Verification items for the finished model (mm, model axes). Face numbers are marked on the shaded views. A direction names the side the tool comes from. Give positions to 0.01 mm unless a question says otherwise; leave off trailing zeros. Write each loop counter-clockwise with the first axis right and the second up, starting at its lowest first coordinate (ties: lowest second). Pieces come first, ordered by that corner, then holes. Notation, with made-up numbers: (-25.75, 79.25) - (-9.75, 79.25) arc R36 ccw to (-9.75, 114.25) - close; hole circle Ø11 at (27, 70.25). An arc over 180 degrees is marked (long way). Answer as a JSON object with one key per item and string values. Group by question number.
Item 1: Scan lines: line 1 along Y through (x, z) = (1312.5, 29); line 2 along X through (y, z) = (-642, 140). Record each from-to range of solid material in increasing order. Write a range as [from, to].
Item 2: Tool access check on the marked faces 1 and 2. Record the directions out of +Z, -Z, +X, -X, +Y, -Y that give a thin tool (end or side, any length) a straight path to the whole face; none if there is none.
Item 3: Sectioned sample at C-C, the plane x = 1124.5. Record the boundary of the cut face in (y, z).
Item 4: Go/stop test with a flat-tipped pin: pin 1 (1.5 mm diameter, centred on y = -639.5, z = 38, fed in from +X). Record where the tip stops, or that it passes through.
Item 5: Sectioned sample at B-B, the plane z = 73.5. Record the boundary of the cut face in (x, y).
Item 6: Sectioned sample at A-A, the plane y = -674.5. Record the boundary of the cut face in (x, z), and give its area (3 significant figures).
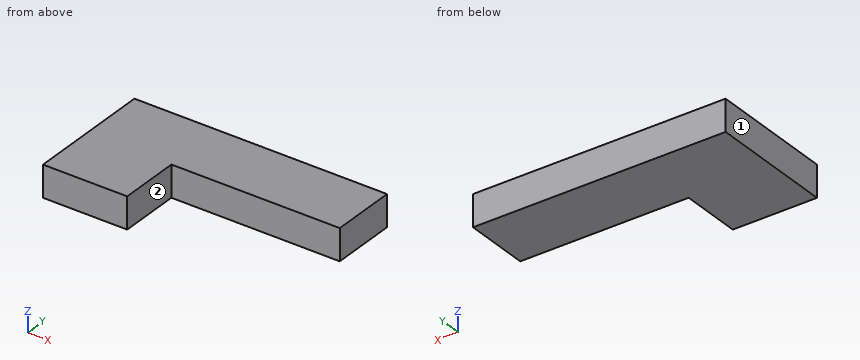
Autodesk Inventor part; units mm, degrees
ref_plane "YZ Plane" through (0, 0, 0) normal (1, 0, 0) x (0, 1, 0)
ref_plane "XZ Plane" through (0, 0, 0) normal (0, 1, 0) x (-1, 0, 0)
ref_plane "XY Plane" through (0, 0, 0) normal (0, 0, 1) x (1, 0, 0)
sketch "Sketch1" plane through (0, 0, 0) normal (0, 0, 1) x (1, 0, 0)
  line L0 (0, 0) -> (1524, 0)
  line L1 (1524, 0) -> (1524, -393.7)
  line L2 (1524, -393.7) -> (508, -393.7)
  line L3 (0, -393.7) -> (0, 0)
  line L4 (0, 0) -> (928.4892, 0)
  line L5 (420.4892, -393.7) -> (508, -393.7)
  line L6 (0, -393.7) -> (0, 0)
  line L7 (0, 0) -> (508, 0)
  line L8 (508, -393.7) -> (508, -762)
  line L9 (508, -762) -> (0, -762)
  line L10 (0, -762) -> (0, 0)
  dimension "d0" = 393.7
  dimension "d1" = 1524
  dimension "d2" = 762
  dimension "d3" = 508
extrude "Extrusion1" add sketch "Sketch1" along normal blind 190.5
properties part number "laser-enclosure"
Geometry check:
{
 "1": {"line 1": "[-393.7, 0]", "line 2": "[0, 508]"},
 "2": {"face 1": "+Z, -Z, -X, +Y, -Y", "face 2": "+Z, -Z, +X, -Y"},
 "3": {"outline": "(-393.7, 0) - (0, 0) - (0, 190.5) - (-393.7, 190.5) - close"},
 "4": {"pin 1": "x = 508"},
 "5": {"outline": "(0, -762) - (508, -762) - (508, -393.7) - (1524, -393.7) - (1524, 0) - (0, 0) - close"},
 "6": {"outline": "(0, 0) - (508, 0) - (508, 190.5) - (0, 190.5) - close", "area": "96,800 mm^2"}
}
